Source: CAD feature listing. Evaluate the final solid. Frame: model axes, mm. Face numbers are marked on the shaded views. A direction names the side the tool comes from. Coordinates: 2 decimals unless noted, no trailing zeros. Loops run counter-clockwise (first coordinate to the right, second up) from the corner with the lowest first, then second, coordinate; pieces in that order, holes last. Notation, with made-up numbers: (-1, -10) -> (46, -10) arc R26 ccw to (46, 19) -> close; hole circle Ø7 at (53, -10.5). An arc over 180 degrees is marked (long way). Answer as a JSON object with one key per item and string values. Group by question number.
from build123d import *

# Parameters (mm, degrees)
SKETCH_1_R      = 10
EXTRUDE_1_DEPTH = 2
SKETCH_2_W      = 50
SKETCH_2_H      = 50
SKETCH_2_R      = 11.5
SKETCH_2_R_2    = 1.51
EXTRUDE_2_DEPTH = 2
SKETCH_3_R      = 1.51
EXTRUDE_3_DEPTH = 2


with BuildPart() as part:
    # 草图1 → 凸台-拉伸1 (new body)
    with BuildSketch(Plane.XY):
        with BuildLine():
            Line((0, 0), (0, 30))
            Line((0, 30), (35.355339059, 65.355339059))
            Line((35.355339059, 65.355339059), (67.781745931, 32.928932188))
            ThreePointArc((67.781745931, 32.928932188), (69.949473444, 29.6846987), (70.710678119, 25.857864376))
            Line((70.710678119, 25.857864376), (70.710678119, 0))
            Line((70.710678119, 0), (0, 0))
        make_face()
        with Locations((45.961940777, 19.393398282)):
            Circle(SKETCH_1_R, mode=Mode.SUBTRACT)
    extrude_1 = extrude(amount=EXTRUDE_1_DEPTH)

    # 草图2 → 凸台-拉伸2 (add)
    with BuildSketch(Plane(origin=(-15, 15, 0), x_dir=(0, 0, 1), z_dir=(-0.7071067811865477, 0.7071067811865475, 0))):
        with Locations((-25, 46.213203436)):
            Rectangle(SKETCH_2_W, SKETCH_2_H)
        with Locations(Location((-25, 46.213203436, 0), (0, 0, 270))):
            Circle(SKETCH_2_R, mode=Mode.SUBTRACT)
        with Locations(Location((-40.5, 61.713203436, 0), (0, 0, 270))):
            Circle(SKETCH_2_R_2, mode=Mode.SUBTRACT)
        with Locations(Location((-9.5, 61.713203436, 0), (0, 0, 270))):
            Circle(SKETCH_2_R_2, mode=Mode.SUBTRACT)
        with Locations(Location((-9.5, 30.713203436, 0), (0, 0, 270))):
            Circle(SKETCH_2_R_2, mode=Mode.SUBTRACT)
        with Locations(Location((-40.5, 30.713203436, 0), (0, 0, 270))):
            Circle(SKETCH_2_R_2, mode=Mode.SUBTRACT)
    extrude(amount=-EXTRUDE_2_DEPTH)

    # 草图3 → 凸台-拉伸3 (add)
    with BuildSketch(Plane.XZ):
        with BuildLine():
            Line((0, 2), (0, 20))
            ThreePointArc((0, 20), (0.585786438, 21.414213562), (2, 22))
            Line((2, 22), (68.710678119, 22))
            ThreePointArc((68.710678119, 22), (70.124891681, 21.414213562), (70.710678119, 20))
            Line((70.710678119, 20), (70.710678119, 2))
            Line((70.710678119, 2), (0, 2))
        make_face()
        with Locations(Location((10, 11, 0), (0, 0, 270))):
            Circle(SKETCH_3_R, mode=Mode.SUBTRACT)
        with Locations(Location((20, 11, 0), (0, 0, 270))):
            Circle(SKETCH_3_R, mode=Mode.SUBTRACT)
        with Locations(Location((30, 11, 0), (0, 0, 270))):
            Circle(SKETCH_3_R, mode=Mode.SUBTRACT)
        with Locations(Location((40, 11, 0), (0, 0, 270))):
            Circle(SKETCH_3_R, mode=Mode.SUBTRACT)
        with Locations(Location((50, 11, 0), (0, 0, 270))):
            Circle(SKETCH_3_R, mode=Mode.SUBTRACT)
        with Locations(Location((60, 11, 0), (0, 0, 270))):
            Circle(SKETCH_3_R, mode=Mode.SUBTRACT)
    extrude_3 = extrude(amount=-EXTRUDE_3_DEPTH)

    # 镜向1: 凸台-拉伸1, 凸台-拉伸3 across plane
    add(extrude_1.mirror(Plane(origin=(0, 0, -25), x_dir=(1, 0, 0), z_dir=(0, 0, -1))))
    add(extrude_3.mirror(Plane(origin=(0, 0, -25), x_dir=(1, 0, 0), z_dir=(0, 0, -1))))


solid = part.part
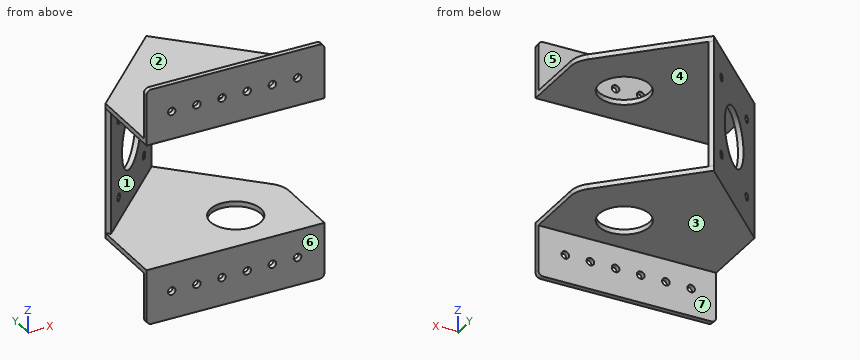
1. Section query D-D on x = 60. Return loops of the section in (y, z), then the cut area to 3 significant figures.
2. Mould query, pull axis Z, two halves, no side actions, for the marked faces 1, 2, 3 and 4. Classes: pulls with the +Z half, pulls with the -Z half, needs draft (parallel to the pull), parting line crosses it, or undercut.
3. Pin query (flat end, axial travel): pin 1 Ø3 at (x, z) = (32.5, -62.5) entering from +Y; pin 2 Ø5 at (x, z) = (23, -16) entering from -Y; pin 3 Ø6 at (x, y) = (61.5, 26) entering from -Z. Return the tip coordinate at first contact, or that it passes through.
4. Section query A-A on z = 11. Return loops of the section in (x, y), then the cut area to 3 significant figures.
5. Section query C-C on y = 11.5. Return loops of the section in (x, z), then the cut area to 3 significant figures.
6. Reachability of the marked faces 5, 6 and 7 from +Z, -Z, +X, -X, +Y, -Y: full face, straight path, thin tool, end or side. Return the list, or none.
7. Section query B-B on x = 40. Return loops of the section in (y, z) (3 decimals), then the cut area to 3 significant figures.
8. Ray query, L1, parallel to Z at x = 16.5, y = 42; L2, parallel to Y at x = 56.5, z = -59; L3, parallel to X at y = 38.5, z = -20. Return the intervals inside material, ascending.
Solved:
{
 "1": {"outline": "(0, -72) -> (2, -72) -> (2, -62.51) -> (0, -62.51) -> close; (0, -59.49) -> (2, -59.49) -> (2, -52) -> (40.71, -52) -> (40.71, -50) -> (0, -50) -> close; (0, 0) -> (40.71, 0) -> (40.71, 2) -> (2, 2) -> (2, 9.49) -> (0, 9.49) -> close; (0, 12.51) -> (2, 12.51) -> (2, 22) -> (0, 22) -> close", "area": "231 mm^2"},
 "2": {"face 1": "undercut", "face 2": "pulls with the +Z half", "face 3": "pulls with the -Z half", "face 4": "undercut"},
 "3": {"pin 1": "y = 2", "pin 2": "y = 48.66", "pin 3": "z = -52"},
 "4": {"outline": "(0, 0) -> (8.49, 0) -> (8.49, 2) -> (0, 2) -> close; (11.51, 0) -> (18.49, 0) -> (18.49, 2) -> (11.51, 2) -> close; (21.51, 0) -> (28.49, 0) -> (28.49, 2) -> (21.51, 2) -> close; (31.51, 0) -> (38.49, 0) -> (38.49, 2) -> (31.51, 2) -> close; (41.51, 0) -> (48.49, 0) -> (48.49, 2) -> (41.51, 2) -> close; (51.51, 0) -> (58.49, 0) -> (58.49, 2) -> (51.51, 2) -> close; (61.51, 0) -> (70.71, 0) -> (70.71, 2) -> (61.51, 2) -> close", "area": "105 mm^2"},
 "5": {"outline": "(0, -52) -> (39.82, -52) -> (39.82, -50) -> (0, -50) -> close; (0, 0) -> (39.82, 0) -> (39.82, 2) -> (0, 2) -> close; (52.1, -52) -> (70.71, -52) -> (70.71, -50) -> (52.1, -50) -> close; (52.1, 0) -> (70.71, 0) -> (70.71, 2) -> (52.1, 2) -> close", "area": "234 mm^2"},
 "6": {"face 5": "+Z, +X, -X, +Y", "face 6": "+Z, -Z, +X, -X, -Y", "face 7": "-Z, +X, -X, +Y"},
 "7": {"outline": "(0, -72) -> (2, -72) -> (2, -62.51) -> (0, -62.51) -> close; (0, -59.49) -> (2, -59.49) -> (2, -52) -> (11.365, -52) -> (11.365, -50) -> (0, -50) -> close; (0, 0) -> (11.365, 0) -> (11.365, 2) -> (2, 2) -> (2, 9.49) -> (0, 9.49) -> close; (0, 12.51) -> (2, 12.51) -> (2, 22) -> (0, 22) -> close; (27.422, -52) -> (60.711, -52) -> (60.711, -50) -> (27.422, -50) -> close; (27.422, 0) -> (60.711, 0) -> (60.711, 2) -> (27.422, 2) -> close", "area": "247 mm^2"},
 "8": {"L1": "-52 to -50, 0 to 2", "L2": "0 to 2", "L3": "8.5 to 11.33"}
}
